Autodesk Inventor part; units mm, degrees
ref_plane "YZ Plane" through (0, 0, 0) normal (1, 0, 0) x (0, 1, 0)
ref_plane "XZ Plane" through (0, 0, 0) normal (0, 1, 0) x (-1, 0, 0)
ref_plane "XY Plane" through (0, 0, 0) normal (0, 0, 1) x (1, 0, 0)
sketch "Sketch1" plane through (0, 0, 0) normal (0, 0, 1) x (1, 0, 0)
  circle A0 centre (0, 0) radius 2.5
  dimension "d0" = 5
extrude "Extrusion1" add sketch "Sketch1" along normal blind 52.5
sketch "Sketch2" plane through (0, 0, 52.5) normal (0, 0, 1) x (1, 0, 0)
  circle A0 centre (0, 0) radius 2.5
  circle A1 centre (0, 0) radius 1.5
  dimension "d3" = 3
extrude "Extrusion2" cut sketch "Sketch2" against normal blind 4.2
chamfer "Chamfer1" distance 0.2 angle 45 3 edges at (-1.5, 0, 52.5) (-2.5, 0, 48.3) (-2.5, 0, 0)
properties part number "SensorKopf_Encoder_Welle" material "Aluminum 6061-AHC"
Model file for the job. Use its own axes, mm. A direction names the side the tool comes from. Give positions to 0.01 mm unless a question says otherwise; leave off trailing zeros. Loops run counter-clockwise (first coordinate to the right, second up) from the corner with the lowest first, then second, coordinate; pieces in that order, holes last. Notation, with made-up numbers: (-24, 11) - (-8, 11) arc R15 ccw to (-8, 40) - close; hole circle Ø1 at (-15.75, 38). An arc over 180 degrees is marked (long way). Use one line per item in the form item = value.
(1) Drop a flat-ended pin along its axis: P1, Ø1, axis at y = -2, z = 29.5, coming from the -X side. Give the stop position or say it passes through.
Determined:
P1 = -2
(2) Cut at A-A (x = 0). Give the cut face in (y, z), then the cut area to 3 significant figures.
Determined:
outline = (-2.5, 0.2) - (-2.3, 0) - (2.3, 0) - (2.5, 0.2) - (2.5, 48.1) - (2.3, 48.3) - (1.5, 48.3) - (1.5, 52.3) - (1.3, 52.5) - (-1.3, 52.5) - (-1.5, 52.3) - (-1.5, 48.3) - (-2.3, 48.3) - (-2.5, 48.1) - close
area = 254 mm^2
(3) 3-axis set-ups, long thin cutter, end or side, ignore diameter. For faces 1 (the face through (0, -2, 48.3)), 2 (the face through (-0.54, 2.44, 23.81)): which of +Z, -Z, +X, -X, +Y, -Y reach the whole face in a straight line?
Determined:
face_1 = +Z
face_2 = +Z, -Z
(4) Cut at C-C (z = 8.5). Give the cut face in (x, y).
Determined:
outline = circle Ø5 at (0, 0)
(5) Pull direction Z, two halves, no side cores. Call faces 3 (the face through (-1.5, 0.07, 50.33)), 4 (the face through (0, 0, 52.5)), 5 (the face through (0, 0, 0)): pulls with the +Z half, pulls with the -Z half, needs draft (parallel to the pull), parting line crosses it, or undercut.
Determined:
face_3 = needs draft
face_4 = pulls with the +Z half
face_5 = pulls with the -Z half
(6) Drill centre lines: L1, parallel to Z at x = 1.7, y = 0.3; L2, parallel to X at y = 2.2, z = 15.5; L3, parallel to X at y = -1.65, z = 46.5. Where is each one in solid material? Low to high.
Determined:
L1 = 0 to 48.3
L2 = -1.19 to 1.19
L3 = -1.88 to 1.88
